```python
from build123d import *

# Parameters (mm, degrees)
SKETCH2_R           = 13.700000032
BOSS_EXTRUDE1_DEPTH = 57.000000046
SKETCH15_OUTSIDE_W  = 43.184
SKETCH15_OUTSIDE_H  = 43.184
SKETCH15_OUTSIDE_R  = 1.143
CUT_EXTRUDE10_DEPTH = 12.900000108
SKETCH18_OUTSIDE_W  = 43.184
SKETCH18_OUTSIDE_H  = 43.184
SKETCH18_OUTSIDE_R  = 4.899999979
CUT_EXTRUDE13_DEPTH = 2.600000134
SKETCH21_OUTSIDE_W  = 43.184
SKETCH21_OUTSIDE_H  = 43.184
SKETCH21_OUTSIDE_R  = 1.099999959
CUT_EXTRUDE16_DEPTH = 1.299999686
SKETCH23_OUTSIDE_W  = 43.184
SKETCH23_OUTSIDE_H  = 43.184
SKETCH23_OUTSIDE_R  = 4.899999979
CUT_EXTRUDE18_DEPTH = 2.200000172


with BuildPart() as part:
    # Sketch2 → Boss-Extrude1 (new body)
    with BuildSketch(Plane(origin=(0, 0, 0), x_dir=(1, 0, 0), z_dir=(0, 1, 0))):
        with Locations(Location((0, 0, 0), (0, 0, 270))):
            Circle(SKETCH2_R)
    extrude(amount=BOSS_EXTRUDE1_DEPTH)

    # Sketch15 outside → Cut-Extrude10 (cut)
    with BuildSketch(Plane(origin=(0, 57.000000046, 0), x_dir=(1, 0, 0), z_dir=(0, 1, 0))):
        Rectangle(SKETCH15_OUTSIDE_W, SKETCH15_OUTSIDE_H)
        with Locations(Location((0, 0, 0), (0, 0, 270))):
            Circle(SKETCH15_OUTSIDE_R, mode=Mode.SUBTRACT)
    extrude(amount=-CUT_EXTRUDE10_DEPTH, mode=Mode.SUBTRACT)

    # Sketch18 outside → Cut-Extrude13 (cut)
    with BuildSketch(Plane(origin=(0, 44.099999938, 0), x_dir=(1, 0, 0), z_dir=(0, 1, 0))):
        Rectangle(SKETCH18_OUTSIDE_W, SKETCH18_OUTSIDE_H)
        with Locations(Location((0, 0, 0), (0, 0, 270))):
            Circle(SKETCH18_OUTSIDE_R, mode=Mode.SUBTRACT)
    extrude(amount=-CUT_EXTRUDE13_DEPTH, mode=Mode.SUBTRACT)

    # Sketch21 outside → Cut-Extrude16 (cut)
    with BuildSketch(Plane(origin=(0, 0, 0), x_dir=(-1, 0, 0), z_dir=(0, -1, 0))):
        Rectangle(SKETCH21_OUTSIDE_W, SKETCH21_OUTSIDE_H)
        with Locations(Location((0, 0, 0), (0, 0, 90))):
            Circle(SKETCH21_OUTSIDE_R, mode=Mode.SUBTRACT)
    extrude(amount=-CUT_EXTRUDE16_DEPTH, mode=Mode.SUBTRACT)

    # Sketch23 outside → Cut-Extrude18 (cut)
    with BuildSketch(Plane.XZ):
        Rectangle(SKETCH23_OUTSIDE_W, SKETCH23_OUTSIDE_H)
        with Locations(Location((0, 0, 0), (0, 0, 90))):
            Circle(SKETCH23_OUTSIDE_R, mode=Mode.SUBTRACT)
    extrude(amount=-CUT_EXTRUDE18_DEPTH, mode=Mode.SUBTRACT)


solid = part.part
```
Geometry check sheet. Reference: the model listing, model coordinates, mm. A direction names the side the tool comes from. Give positions to 0.01 mm unless a question says otherwise; leave off trailing zeros. Order: outer loops, then holes, each group sorted by start corner. A loop starts at its lowest first (then second) coordinate and runs counter-clockwise, first axis right, second up. Notation, with made-up numbers: (79, -5.75) - (86, -5.75) arc R12 cw to (86, -0.75) - close; hole circle Ø4 at (-6, 50.25). An arc over 180 degrees is marked (long way). Write item = value, one per line. Start each with the question number.
1) Gauge pin test, flat ends, axial feed: pin 1 Ø1.5 at (x, y) = (4.5, 44.5) entering from +Z; pin 2 Ø8 at (x, z) = (1, 2.5) entering from +Y; pin 3 Ø2 at (x, z) = (5, -6.5) entering from -Y; pin 4 Ø1 at (x, z) = (-3.5, -1) entering from -Y. Record the tip position at first contact, or that the pin passes through.
2) Scan lines: L1, parallel to Y at x = -6.5, z = 9.5; L2, parallel to X at y = 42.5, z = 0; L3, parallel to X at y = 26.5, z = -6.5. Record each from-to range of solid material in increasing order.
3) Section check A-A (x = 0). Enter the section's corners in (y, z), then the cut area to 3 significant figures.
4) Section check C-C (y = 31). Enter the section's corners in (x, z), then the cut area to 3 significant figures.
5) Section check B-B (z = -1.75). Enter the section's corners in (x, y), then the cut area to 3 significant figures.
6) Access from +Z, -Z, +X, -X, +Y, -Y to the whole of each face (thin tool, end or side, straight path). Record for faces 1 (the cylindrical face through (1.09, 0.64, 0.14)), 2 (the cylindrical face through (-13.374, 21.575, -2.97)), 3 (the cylindrical face through (4.132, 42.818, 2.634)).
7) Section check D-D (x = 4). Enter the section's corners in (y, z).
Geometry check:
q1.pin_1 = 3.01
q1.pin_2 = 57
q1.pin_3 = 2.2
q1.pin_4 = 1.3
q2.L1 = 2.2 to 41.5
q2.L2 = -4.9 to 4.9
q2.L3 = -12.06 to 12.06
q3.outline = (0, -1.1) - (1.3, -1.1) - (1.3, -4.9) - (2.2, -4.9) - (2.2, -13.7) - (41.5, -13.7) - (41.5, -4.9) - (44.1, -4.9) - (44.1, -1.14) - (57, -1.14) - (57, 1.14) - (44.1, 1.14) - (44.1, 4.9) - (41.5, 4.9) - (41.5, 13.7) - (2.2, 13.7) - (2.2, 4.9) - (1.3, 4.9) - (1.3, 1.1) - (0, 1.1) - close
q3.area = 1,140 mm2
q4.outline = circle Ø27.4 at (0, 0)
q4.area = 590 mm2
q5.outline = (-13.59, 2.2) - (-4.58, 2.2) - (-4.58, 1.3) - (4.58, 1.3) - (4.58, 2.2) - (13.59, 2.2) - (13.59, 41.5) - (4.58, 41.5) - (4.58, 44.1) - (-4.58, 44.1) - (-4.58, 41.5) - (-13.59, 41.5) - close
q5.area = 1,100 mm2
q6.face_1 = -Y
q6.face_2 = +Y, -Y
q6.face_3 = +Y
q7.outline = (1.3, -2.83) - (2.2, -2.83) - (2.2, -13.1) - (41.5, -13.1) - (41.5, -2.83) - (44.1, -2.83) - (44.1, 2.83) - (41.5, 2.83) - (41.5, 13.1) - (2.2, 13.1) - (2.2, 2.83) - (1.3, 2.83) - close
